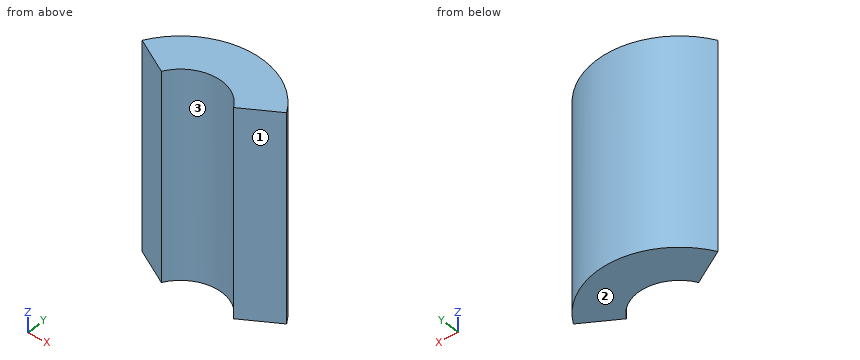
from build123d import *

# Parameters (mm, degrees)
CYLINDER018_W               = 2
CYLINDER018_H               = 10
CYLINDER018_ANGLE           = 120
CYLINDER018_PLACEMENT_ANGLE = 30
CYLINDER016_W               = 4
CYLINDER016_H               = 10
CYLINDER016_ANGLE           = 120
CYLINDER016_PLACEMENT_ANGLE = 30


with BuildPart() as cilindro009:
    # Cylinder018 → Cylinder018 (revolve)
    with BuildSketch(Plane.XZ):
        with Locations((1, 5)):
            Rectangle(CYLINDER018_W, CYLINDER018_H)
    revolve(axis=Axis((0, 0, 0), (0, 0, 1)), revolution_arc=CYLINDER018_ANGLE)


with BuildPart() as cilindro009_1:
    # Cylinder018 placement: moved
    add(cilindro009.part.moved(Location((-30.75, -30, 0))).rotate(Axis((-30.75, -30, 0), (0, 0, 1)), CYLINDER018_PLACEMENT_ANGLE))


with BuildPart() as obj1:
    # Cylinder016 → Cylinder016 (revolve)
    with BuildSketch(Plane.XZ):
        with Locations((2, 5)):
            Rectangle(CYLINDER016_W, CYLINDER016_H)
    revolve(axis=Axis((0, 0, 0), (0, 0, 1)), revolution_arc=CYLINDER016_ANGLE)


with BuildPart() as obj1_1:
    # Cylinder016 placement: moved
    add(obj1.part.moved(Location((-30.75, -30, 0))).rotate(Axis((-30.75, -30, 0), (0, 0, 1)), CYLINDER016_PLACEMENT_ANGLE))

    # Cut007: cut Cilindro009
    add(cilindro009_1.part, mode=Mode.SUBTRACT)


solid = obj1_1.part
Geometry: final body of the model. Coordinates: model frame, mm. Face numbers are marked on the shaded views. Round coordinates to 2 decimals unless told otherwise and drop trailing zeros. Loops run counter-clockwise (first coordinate to the right, second up) from the corner with the lowest first, then second, coordinate; pieces in that order, holes last. Notation, with made-up numbers: M 54.5,-14.75 L 111.5,-14.75 A10 ccw 111.5,0.25 Z; hole C 4,43.25 d10. An arc over 180 degrees is marked long. Put each result on its own line as item: value. Start each with the question number.
(1) Section query B-B (z = 6.75). Return loops of the section in (x, y), then the cut area to 3 significant figures.
(2) Draft query along X for the marked faces 1, 2 and 3. Return one class per face: +X half, -X half, draft (parallel to the pull), parting line (faces both ways), or undercut.
(3) Material intervals for line 1 along X through (y, z) = (-28.8, 5); line 2 along X through (y, z) = (-28.3, 3.5); line 3 along Y through (x, z) = (-28.25, 2.5), sorted ascending. Write a range as [from, to].
(4) Contact query for flat-ended pins moving along their axis: pin 1 Ø2 at (x, z) = (-29, 4.5) entering from +Y; pin 2 Ø1.5 at (y, z) = (-28.5, 5) entering from -X; pin 3 Ø1.5 at (y, z) = (-28.5, 9) entering from +X. Output: stop coordinate, or through.
(5) Section query A-A (y = -28.2). Return loops of the section in (x, z), then the cut area to 3 significant figures.
(6) Section query C-C (x = -30.75). Return loops of the section in (y, z).
Findings below:
1. outline: M -34.21,-28 L -32.48,-29 A2 cw -29.02,-29 L -27.29,-28 A4 ccw Z
1. area: 12.6 mm2
2. face 1: +X half
2. face 2: draft
2. face 3: undercut
3. line 1: x = [-32.83, -32.35], [-29.15, -28.67]
3. line 2: x = [-33.69, -31.8], [-29.7, -27.81]
3. line 3: y = [-28.56, -26.88]
4. pin 1: stops at y = -26.07
4. pin 2: stops at x = -34.21
4. pin 3: stops at x = -27.29
5. outline: M -33.87,0 L -31.62,0 L -31.62,10 L -33.87,10 Z; M -29.88,0 L -27.63,0 L -27.63,10 L -29.88,10 Z
5. area: 44.9 mm2
6. outline: M -28,0 L -26,0 L -26,10 L -28,10 Z
